Can you work these out from the drawing? Everything is in mm from the part's minimum corner. Round coordinates to 2 decimals unless told otherwise and drop trailing zeros. Loops run counter-clockwise (first coordinate to the right, second up) from the corner with the lowest first, then second, coordinate; pieces in that order, holes last. Notation, with made-up numbers: (16, 28) - (20, 28) arc R19 cw to (20, 32) - close; hole circle Ø4 at (0.5, -39.75). An arc over 180 degrees is marked (long way). Answer as a JSON object with one key per item and string values. Group by question number.
1) I want a section at D-D, the plane y = 3.6. Please give me the cut outline in (x, z) (1 decimal).
2) I want a section at B-B, the plane z = 6. Please give me the cut outline in (x, y) (1 decimal).
3) I want a section at A-A, the plane x = 7.5. Please give me the cut outline in (y, z) (1 decimal).
4) I want a section at C-C, the plane y = 1.7. Please give me the cut outline in (x, z) (1 decimal).
5) Will these pins go through, and if not, where does the flat tip stop? P1, Ø1.5, axis at x = 26, y = 2, coming from the +Z side; P2, Ø1, axis at x = 5, z = 4.5, coming from the -Y side.
6) If I drill on line 1 along X through (y, z) = (3.05, 7) (1 decimal); line 2 along X through (y, z) = (2.95, 8.25) (1 decimal); line 3 along Z through (x, y) = (38.5, 2.1), over which ranges is the centre line in solid material (lowest first)? Write a range as [from, to].
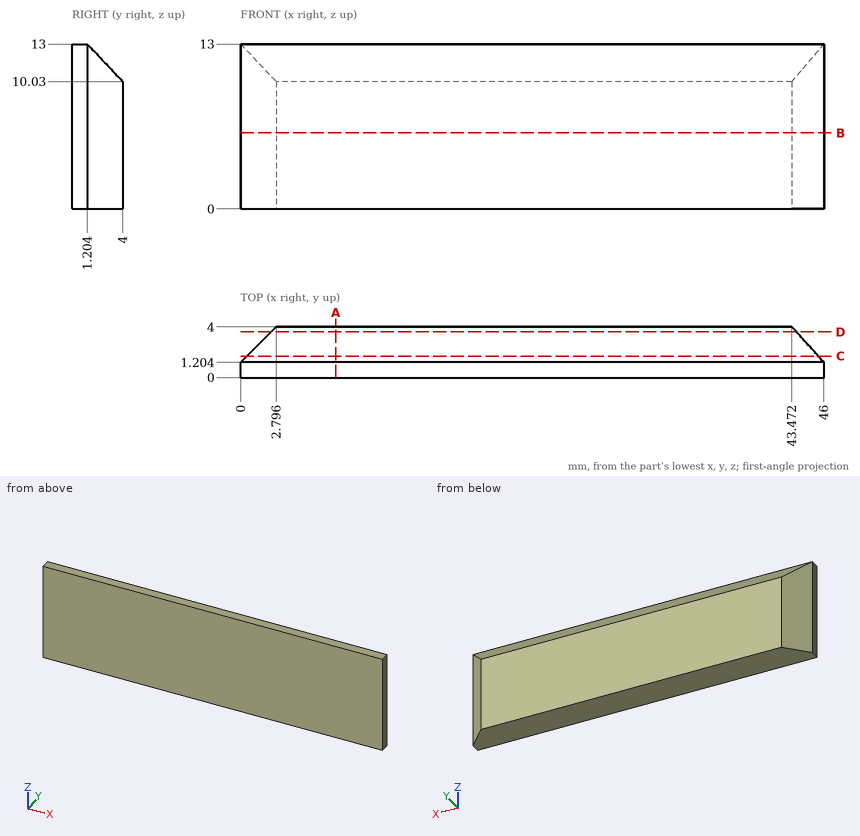
Outcome:
{
 "1": {"outline": "(2.4, 0) - (43.8, 0) - (43.8, 10.5) - (2.4, 10.5) - close"},
 "2": {"outline": "(0, 0) - (46, 0) - (46, 1.2) - (43.5, 4) - (2.8, 4) - (0, 1.2) - close"},
 "3": {"outline": "(0, 0) - (4, 0) - (4, 10) - (1.2, 13) - (0, 13) - close"},
 "4": {"outline": "(0.5, 0) - (45.6, 0) - (45.6, 12.5) - (0.5, 12.5) - close"},
 "5": {"P1": "z = 12.95", "P2": "y = 0"},
 "6": {"line 1": "[1.8, 44.3]", "line 2": "[1.7, 44.4]", "line 3": "[0, 12.05]"}
}
